Check sheet for the modelled part. Datum: model origin and axes. Units: mm. A direction names the side the tool comes from. Coordinates: 2 decimals unless noted, no trailing zeros. Loops run counter-clockwise (first coordinate to the right, second up) from the corner with the lowest first, then second, coordinate; pieces in that order, holes last. Notation, with made-up numbers: (35, 72.25) -> (91, 72.25) arc R21 ccw to (91, 110.25) -> close; hole circle Ø1 at (60, 51). An arc over 180 degrees is marked (long way). Use CSV: the item, a comma, the result in double quotes.
Autodesk Inventor part; units mm, degrees
ref_plane "YZ Plane" through (0, 0, 0) normal (1, 0, 0) x (0, 1, 0)
ref_plane "XZ Plane" through (0, 0, 0) normal (0, 1, 0) x (-1, 0, 0)
ref_plane "XY Plane" through (0, 0, 0) normal (0, 0, 1) x (1, 0, 0)
sketch "Sketch1" plane through (0, 0, 0) normal (0, 1, 0) x (-1, 0, 0)
  line L0 (0, -55.88) -> (-12.7, -55.88)
  line L1 (-12.7, -36.83) -> (0, -36.83)
  line L2 (0, -36.83) -> (0, -55.88)
  line L3 (-12.7, -55.88) -> (-12.7, -36.83)
  dimension "d1" = 19.05
  dimension "d2" = 12.7
extrude "Extrusion1" add sketch "Sketch1" along normal blind 1.5
sketch "Sketch2" plane through (0, 1.5, 0) normal (0, 1, 0) x (1, 0, 0)
  line L0 (12.7, 36.83) -> (12.7, 55.88)
  line L1 (12.7, 0) -> (10.16, 0)
  circle A0 centre (10.16, 39.37) radius 1.092
  circle A1 centre (10.16, 53.34) radius 1.092
  line L2 (10.16, 53.34) -> (10.16, 39.37)
  point P0 (0, 0)
  dimension "d8" = 2.184
  dimension "d10" = 2.184
  dimension "d71" = 13.97
extrude "Extrusion2" cut sketch "Sketch2" against normal blind 1.5
sketch "Sketch5" plane through (0, 0, -36.83) normal (0, 0, 1) x (1, 0, 0)
  line L0 (12.7, 0) -> (0, 0)
  line L1 (6.35, 0) -> (6.35, 1.5)
  line L2 (12.7, 1.5) -> (0, 1.5)
  line L3 (0, 0) -> (0, 1.5)
  line L4 (0, 0.75) -> (12.7, 0.75)
  line L5 (12.7, 0) -> (12.7, 1.5)
  circle A0 centre (6.35, 0.75) radius 5.175
  dimension "d30" = 10.35
extrude "Extrusion5" add sketch "Sketch5" along normal blind 2 contours A0 L0 | L0 L1 L4 A0 | L0 A0 L4 L1 | L4 L1 L2 A0 | L4 A0 L2 L1 | L2 A0
sketch "Sketch6" plane through (6.35, 0.75, -34.83) normal (0, 0, 1) x (1, 0, 0)
  circle A0 centre (0, 0) radius 5.175
  circle A1 centre (0, 0) radius 3.175
  point P0 (-6.35, -0.75)
  dimension "d35" = 6.35
extrude "Extrusion6" add sketch "Sketch6" along normal blind 9
sketch "Sketch7" plane through (12.7, 0, -55.88) normal (0, 0, -1) x (-1, 0, 0)
  line L0 (0, 0) -> (0, 1.5)
  line L1 (0, 0.75) -> (12.7, 0.75)
  line L2 (12.7, 0) -> (12.7, 1.5)
  line L3 (11.4704, 1.5) -> (1.2296, 1.5)
  line L4 (6.35, 1.5) -> (6.35, 0)
  circle A0 centre (6.35, 0.75) radius 5.175
extrude "Extrusion7" add sketch "Sketch7" along normal blind 2
sketch "Sketch8" plane through (6.35, 0.75, -57.88) normal (0, 0, -1) x (-1, 0, 0)
  circle A0 centre (0, 0) radius 5.175
  circle A1 centre (0, 0) radius 3.175
  point P0 (6.35, -0.75)
  dimension "d40" = 6.35
extrude "Extrusion8" add sketch "Sketch8" along normal blind 9
thread "Thread1"
thread "Thread2"
sketch "Sketch9" plane through (0, 0, -36.83) normal (0, 0, -1) x (-1, 0, 0)
  arc A0 (-11.4704, 0) -> (-1.2296, 0) centre (-6.35, 0.75) ccw
  line L0 (0, 0) -> (-1.2296, 0)
  line L1 (-11.4704, 0) -> (-1.2296, 0)
  circle A1 centre (-6.35, 0.75) radius 5.175
extrude "Extrusion9" add sketch "Sketch9" along normal up to next contours L1 A0
sketch "Sketch10" plane through (10.16, 0, -39.37) normal (0, 1, 0) x (1, 0, 0)
  circle A0 centre (0, 0) radius 1.092
  circle A1 centre (0, 13.97) radius 1.092
  circle A2 centre (0, 13.97) radius 1.092
  point P0 (-10.16, -39.37)
  dimension "d60" = 2.184
extrude "Extrusion10" cut sketch "Sketch10" against normal up to next
sketch "Sketch12" plane through (0, 1.5, 0) normal (0, 1, 0) x (1, 0, 0)
  circle A0 centre (10.16, 39.37) radius 1.092
  circle A1 centre (10.16, 39.37) radius 1.092
  circle A2 centre (10.16, 39.37) radius 2.2225
  circle A3 centre (10.16, 53.34) radius 1.092
  circle A4 centre (10.16, 53.34) radius 1.092
  circle A5 centre (10.16, 53.34) radius 2.2225
  point P0 (0, 0)
  dimension "d54" = 4.445
  dimension "d55" = 4.445
extrude "Extrusion11" cut sketch "Sketch12" against normal blind 5.925
sketch "Sketch13" plane through (0, 1.5, 0) normal (0, 1, 0) x (1, 0, 0)
  line L0 (12.7, 36.83) -> (12.7, 55.88)
  line L1 (12.7, 55.88) -> (0, 55.88)
  line L2 (0, 55.88) -> (0, 36.83)
  line L3 (12.7, 36.83) -> (12.7, 55.88)
  circle A0 centre (10.16, 53.34) radius 1.092
  circle A1 centre (10.16, 53.34) radius 1.092
  line L4 (10.16, 53.34) -> (10.16, 39.37)
  circle A2 centre (10.16, 39.37) radius 1.092
  line L5 (0, 36.83) -> (12.7, 36.83)
  point P0 (0, 0)
  point P1 (12.7, 0)
  dimension "d72" = 13.97
  dimension "d73" = 2.184
extrude "Extrusion12" add sketch "Sketch13" along normal blind 10.4375 contours L5 L2 L1 L0 | A2
thread "Thread6"
sketch "Sketch14" plane through (10.16, 1.5, -53.34) normal (0, -1, 0) x (1, 0, 0)
  circle A0 centre (0, 0) radius 1.092
  circle A1 centre (0, 0) radius 2.2225
  circle A2 centre (0, 13.97) radius 2.2225
  circle A3 centre (0, 13.97) radius 2.2225
  circle A4 centre (0, 0) radius 1.092
  circle A5 centre (0, 13.97) radius 1.092
  point P0 (-10.16, 53.34)
extrude "Extrusion13" cut sketch "Sketch14" against normal blind 1
sketch "Sketch15" plane through (10.16, 1.5, -39.37) normal (0, -1, 0) x (1, 0, 0)
  circle A0 centre (0, 0) radius 1.092
  point P0 (-10.16, 39.37)
extrude "Extrusion14" cut sketch "Sketch15" against normal through all
thread "Thread7"
sketch "Sketch16" plane through (0, 11.9375, 0) normal (0, 1, 0) x (1, 0, 0)
  line L0 (11.525, 36.83) -> (1.175, 36.83)
  line L1 (3.175, 34.83) -> (9.525, 34.83)
  line L2 (1.921, 36.83) -> (6.461, 36.83)
  line L3 (6.461, 36.83) -> (6.961, 36.83)
  line L4 (6.961, 36.83) -> (6.961, 39.854)
  line L5 (6.961, 39.854) -> (1.421, 39.854)
  line L6 (1.421, 39.854) -> (1.421, 36.83)
  line L7 (1.421, 36.83) -> (1.921, 36.83)
  point P0 (0, 0)
  point P1 (0, 36.83)
  point P2 (1.2296, 36.83)
  point P3 (11.4704, 36.83)
  dimension "d114" = 0.5
  dimension "d115" = 3.024
  dimension "d116" = 5.54
extrude "Extrusion15" cut sketch "Sketch16" against normal blind 5
sketch "Sketch17" plane through (0, 11.9375, 0) normal (0, 1, 0) x (1, 0, 0)
  line L0 (12.7, 36.83) -> (12.7, 55.88)
  line L1 (12.7, 55.88) -> (0, 55.88)
  line L2 (0, 36.83) -> (12.7, 36.83)
  line L3 (0, 36.83) -> (12.7, 36.83)
  line L4 (12.7, 36.83) -> (12.7, 55.88)
  line L5 (12.7, 55.88) -> (0, 55.88)
  line L6 (0, 55.88) -> (0, 36.83)
  line L7 (11.4704, 41.1651) -> (11.4704, 51.5449)
  line L8 (11.43, 42.545) -> (12.43, 42.545) construction
  line L9 (11.43, 50.165) -> (12.43, 50.165) construction
  line L10 (12.7, 41.545) -> (12.7, 51.165)
  line L11 (12.7, 41.545) -> (12.7, 41.045)
  line L12 (12.7, 41.045) -> (9.93, 41.045)
  line L13 (9.93, 41.045) -> (9.93, 51.665)
  line L14 (9.93, 51.665) -> (12.7, 51.665)
  line L15 (12.7, 51.165) -> (12.7, 51.665)
  point P0 (0, 0)
  dimension "d110" = 2.77
  dimension "d111" = 10.62
  dimension "d112" = 90
extrude "Extrusion16" cut sketch "Sketch17" against normal blind 8 contours L12 L13 L14 L0
properties part number "Line Sensor 6 Bracket"
1) Access from +Z, -Z, +X, -X, +Y, -Y to the whole of each face (thin tool, end or side, straight path). Record for faces 4 (the flat face through (6, 1, -34.83)), 5 (the flat face through (11, 8, -51.665)), 6 (the cylindrical face through (7.94, -0.05, -53.44)).
Answer below:
face 4,"+Z"
face 5,"+X, +Y"
face 6,"-Y"
2) Cross-section at D-D on x = 6.5. Record the boundary of the cut face in (y, z).
Answer below:
outline,"(-4.42, -66.88) -> (-2.42, -66.88) -> (-2.42, -57.88) -> (3.92, -57.88) -> (3.92, -66.88) -> (5.92, -66.88) -> (5.92, -55.88) -> (11.94, -55.88) -> (11.94, -39.85) -> (6.94, -39.85) -> (6.94, -36.83) -> (5.92, -36.83) -> (5.92, -25.83) -> (3.92, -25.83) -> (3.92, -34.83) -> (-2.42, -34.83) -> (-2.42, -25.83) -> (-4.42, -25.83) -> (-4.42, -55.88) -> close"
3) Go/stop test with flat-tipped pins: pin 1 Ø3.5 at (x, z) = (4.5, -38) entering from +Y; pin 2 Ø3 at (x, z) = (10.16, -39.37) entering from -Y; pin 3 Ø3 at (x, y) = (6.5, 0.5) entering from +Z. Record where each tip stops, or that it passes through.
Answer below:
pin 1,"stops at y = 6.94"
pin 2,"stops at y = 2.5"
pin 3,"stops at z = -34.83"
4) Cross-section at B-B on y = 9. Record the boundary of the cut face in (x, z) (3 decimals), and give its area (3 significant figures).
Answer below:
outline,"(0, -55.88) -> (12.7, -55.88) -> (12.7, -51.665) -> (9.93, -51.665) -> (9.93, -41.045) -> (12.7, -41.045) -> (12.7, -36.83) -> (6.961, -36.83) -> (6.961, -39.854) -> (1.421, -39.854) -> (1.421, -36.83) -> (0, -36.83) -> close; hole circle Ø2.184 at (10.16, -53.34); hole circle Ø2.184 at (10.16, -39.37)"
area,"188 mm²"
5) Cross-section at A-A on z = -39.37. Record the boundary of the cut face in (x, y), and give its area (3 significant figures).
Answer below:
outline,"(0, 0) -> (1.23, 0) arc R5.18 ccw to (7.94, -4.18) -> (7.94, 2.5) -> (9.07, 2.5) -> (9.07, 11.94) -> (6.96, 11.94) -> (6.96, 6.94) -> (1.42, 6.94) -> (1.42, 11.94) -> (0, 11.94) -> close; (11.25, 2.5) -> (12.38, 2.5) -> (12.38, 0) -> (12.7, 0) -> (12.7, 11.94) -> (11.25, 11.94) -> close"
area,"116 mm²"
6) Thickness scan on line 1 along Y through (x, z) = (6.35, -31.75) (3 decimals); line 2 along Z through (x, y) = (10.16, 5) (3 decimals); line 3 along Z through (x, y) = (11, 6.5) (3 decimals). Record the ranges inside material, lowest first. Write a range as from..to.
Answer below:
line 1,"y = -4.425..-2.425, 3.925..5.925"
line 2,"z = -55.88..-54.432, -52.248..-51.665, -41.045..-40.462, -38.278..-36.83"
line 3,"z = -55.88..-54.038, -52.642..-51.665, -41.045..-40.068, -38.672..-36.83"
7) Cross-section at C-C on z = -53.34. Record the boundary of the cut face in (x, y), and give its area (3 significant figures).
Answer below:
outline,"(0, 0) -> (1.23, 0) arc R5.18 ccw to (7.94, -4.18) -> (7.94, 2.5) -> (9.07, 2.5) -> (9.07, 11.94) -> (0, 11.94) -> close; (11.25, 2.5) -> (12.38, 2.5) -> (12.38, 0) -> (12.7, 0) -> (12.7, 11.94) -> (11.25, 11.94) -> close"
area,"144 mm²"
8) Draft check along Z on faces 1 (the flat face through (5, 11.938, -46)), 2 (the flat face through (8, 7, -36.83)), 3 (the cylindrical face through (7.94, -0.05, -39.47)). Enter one of: released by +Z, released by -Z, zero draft, split by the parting line, or undercut.
Answer below:
face 1,"zero draft"
face 2,"released by +Z"
face 3,"undercut"
